Geometry: final body of the model. Coordinates: model frame, mm. Face numbers are marked on the shaded views. Coordinates: 2 decimals unless noted, no trailing zeros. Loops run counter-clockwise (first coordinate to the right, second up) from the corner with the lowest first, then second, coordinate; pieces in that order, holes last. Notation, with made-up numbers: M 42,-30 L 54,-30 A19 cw 54,6 Z; hole C 61,87 d10. An arc over 180 degrees is marked long. Write item = value, one per line. Start each with the question number.
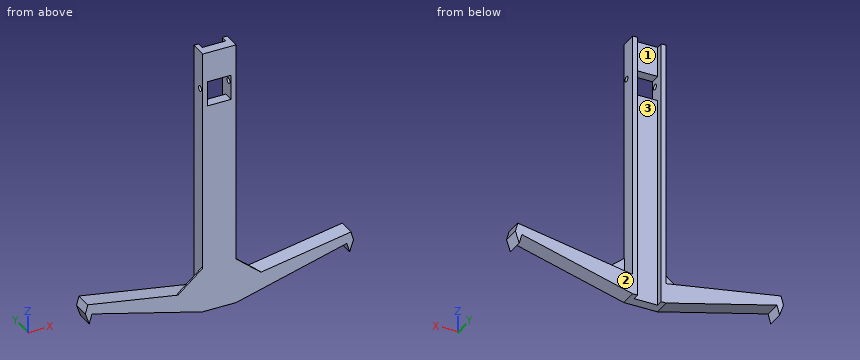
```python
from build123d import *

# Parameters (mm, degrees)
BOSS_EXTRUDE1_DEPTH     = 10
SKETCH2_W               = 14
SKETCH2_H               = 160
CUT_EXTRUDE1_DEPTH      = 4
BOSS_EXTRUDE2_DEPTH     = 10
SKETCH4_W               = 14
SKETCH4_H               = 15
CUT_EXTRUDE2_DEPTH      = 10
CUT_EXTRUDE3_DEPTH      = 20
CUT_EXTRUDE3_DEPTH_BACK = 10
SKETCH5_R               = 1.65
BOSS_EXTRUDE3_DEPTH     = 1


with BuildPart() as part:
    # Sketch1 → Boss-Extrude1 (new body)
    with BuildSketch(Plane(origin=(0, 0, 0), x_dir=(1, 0, 0), z_dir=(0, 1, 0))):
        Polygon((-10, 80), (-80, 61.24355653), (-78.570648621, 55.909144563), (-10, 68), (-10, -80), (10, -80), (10, 68), (78.570648621, 55.909144563), (80, 61.24355653), (10, 80), align=None)
    extrude(amount=BOSS_EXTRUDE1_DEPTH)

    # Sketch2 → Cut-Extrude1 (cut)
    with BuildSketch(Plane(origin=(0, 10, 0), x_dir=(1, 0, 0), z_dir=(0, 1, 0))):
        Rectangle(SKETCH2_W, SKETCH2_H)
    extrude(amount=-CUT_EXTRUDE1_DEPTH, mode=Mode.SUBTRACT)

    # Sketch3 → Boss-Extrude2 (add)
    with BuildSketch(Plane(origin=(0, 10, 0), x_dir=(1, 0, 0), z_dir=(0, 1, 0))):
        Polygon((77.689210965, 68.074387668), (76.136296695, 62.27883271), (80, 61.24355653), align=None)
        Polygon((-77.689210965, 68.074387668), (-76.136296695, 62.27883271), (-80, 61.24355653), align=None)
    extrude(amount=-BOSS_EXTRUDE2_DEPTH)

    # Sketch4 → Cut-Extrude2 (cut)
    with BuildSketch(Plane(origin=(0, 6, 0), x_dir=(1, 0, 0), z_dir=(0, 1, 0))):
        with Locations((0, -54.5)):
            Rectangle(SKETCH4_W, SKETCH4_H)
    extrude(amount=-CUT_EXTRUDE2_DEPTH, mode=Mode.SUBTRACT)

    # Sketch5 → Cut-Extrude3 (cut, two sides: drawn at the far end of the back side and taken through both)
    with BuildSketch(Plane.ZY.offset(-7).offset(-CUT_EXTRUDE3_DEPTH_BACK)):
        with Locations(Location((57, 3, 0), (0, 0, 180))):
            Circle(SKETCH5_R)
    extrude(amount=CUT_EXTRUDE3_DEPTH + CUT_EXTRUDE3_DEPTH_BACK, mode=Mode.SUBTRACT)

    # Sketch6 → Boss-Extrude3 (add)
    with BuildSketch(Plane.XZ):
        Polygon((-24.772116295, -65.395277335), (-10, -53), (-10, -68), align=None)
        Polygon((10, -53), (24.772116295, -65.395277335), (10, -68), align=None)
    extrude(amount=-BOSS_EXTRUDE3_DEPTH)


solid = part.part
```
Item 1: Section query C-C (x = 37). Return the cut outline in (y, z), plus the area to 3 significant figures.
Item 2: Line query: line 1 (X direction, y = 8.25, z = -15); line 2 (Y direction, x = -8, z = 57); line 3 (Z direction, x = -6, y = 4.5). Output: solid intervals per line, ascending. Write a range as from..to.
Item 3: First-contact query: pin 1 (4.5 mm diameter, centred on y = 3, z = 57, fed in from +X); pin 2 (11 mm diameter, centred on x = -1, z = 68.5, fed in from +Y); pin 3 (5 mm diameter, centred on x = 62, y = 7, fed in from +Z); pin 4 (16 mm diameter, centred on x = 17.5, z = -61, fed in from +Y). Flat tips, straight axial feed; report the tip coordinate or a pass-through.
Item 4: Pull-direction query (X, two-part tool) for the marked faces 1, 2 and 3; classes: released by +X, released by -X, zero draft, split by the parting line, or undercut.
Item 5: Section query A-A (y = 3). Return the cut outline in (x, z), plus the area to 3 significant figures.
Item 6: Section query D-D (x = 55). Return the cut outline in (y, z), plus the area to 3 significant figures.
Item 7: Section query B-B (z = 70). Return the cut outline in (x, y).
Verdict:
q1.outline = M 0,-72.77 L 10,-72.77 L 10,-63.24 L 0,-63.24 Z
q1.area = 95.3 mm2
q2.line_1 = -10..-7, 7..10
q2.line_2 = 0..1.35, 4.65..10
q2.line_3 = -80..47, 62..80
q3.pin_1 = 10
q3.pin_2 = 6
q3.pin_3 = -58.39
q3.pin_4 = 10
q4.face_1 = undercut
q4.face_2 = zero draft
q4.face_3 = undercut
q5.outline = M -80,-61.24 L -77.69,-68.07 L -76.14,-62.28 L -10,-80 L 10,-80 L 76.14,-62.28 L 77.69,-68.07 L 80,-61.24 L 78.57,-55.91 L 10,-68 L 10,55.35 L 7,55.35 L 7,47 L -7,47 L -7,55.35 L -10,55.35 L -10,-68 L -78.57,-55.91 Z; M -10,58.65 L -7,58.65 L -7,62 L 7,62 L 7,58.65 L 10,58.65 L 10,80 L -10,80 Z
q5.area = 4,220 mm2
q6.outline = M 0,-67.94 L 10,-67.94 L 10,-60.07 L 0,-60.07 Z
q6.area = 78.8 mm2
q7.outline = M -10,0 L 10,0 L 10,10 L 7,10 L 7,6 L -7,6 L -7,10 L -10,10 Z
